Autodesk Inventor part; units mm, degrees
ref_plane "YZ Plane" through (0, 0, 0) normal (1, 0, 0) x (0, 1, 0)
ref_plane "XZ Plane" through (0, 0, 0) normal (0, 1, 0) x (-1, 0, 0)
ref_plane "XY Plane" through (0, 0, 0) normal (0, 0, 1) x (1, 0, 0)
sketch "Sketch1" plane through (0, 0, 0) normal (0, 1, 0) x (-1, 0, 0)
  line L0 (0, 0) -> (-25, 0)
  line L1 (-25, 0) -> (-25, -46.5)
  line L2 (-25, -46.5) -> (0, -46.5)
  line L3 (0, -46.5) -> (0, 0)
  dimension "d0" = 25
  dimension "d1" = 46.5
extrude "Extrusion1" add sketch "Sketch1" along normal blind 2
sketch "Sketch2" plane through (0, 2, 0) normal (0, 1, 0) x (1, 0, 0)
  line L0 (25, 46.5) -> (0, 46.5)
  line L1 (0, 46.5) -> (6, 46.5)
  line L2 (6, 46.5) -> (6, 36.5)
  line L3 (6, 36.5) -> (0, 36.5)
  line L4 (0, 36.5) -> (0, 46.5)
  line L5 (25, 46.5) -> (19, 46.5)
  line L6 (19, 46.5) -> (19, 36.5)
  line L7 (19, 36.5) -> (25, 36.5)
  line L8 (25, 36.5) -> (25, 46.5)
  point P0 (0, 0)
  dimension "d4" = 6
  dimension "d5" = 10
  dimension "d6" = 6
extrude "Extrusion2" add sketch "Sketch2" along normal blind 3
sketch "Sketch4" plane through (0, 2, 0) normal (0, 1, 0) x (1, 0, 0)
  line L0 (0, 0) -> (25, 0)
  line L1 (25, 0) -> (25, 36.5)
  point P0 (12.5, 4)
  dimension "d18" = 4
  dimension "d19" = 12.5
hole "Hole2" at (12.5, 2, -4) direction (0, -1, 0) diameter 3.2 end through all
properties part number "mlx_mount_3mm"
For this review, take the finished solid that the model builds, in its own axes (mm). A direction names the side the tool comes from. Round coordinates to 2 decimals unless told otherwise and drop trailing zeros. Write each loop counter-clockwise with the first axis right and the second up, starting at its lowest first coordinate (ties: lowest second). Pieces come first, ordered by that corner, then holes. Notation, with made-up numbers: (22.25, 24.5) -> (43.25, 24.5) arc R26 ccw to (43.25, 63.5) -> close; hole circle Ø8 at (76.25, 88.5). An arc over 180 degrees is marked (long way). One line per question, with ' | ' between items. Start each with the question number.
1) Machinability: for faces 1 (the flat face through (22, 3, -36.5)), 2 (the flat face through (12, 1, 0)), 3 (the flat face through (19, 3, -42)), which of the approach directions +Z, -Z, +X, -X, +Y, -Y give a long, thin tool a straight path to every point of the face, cutting with its end or side? Answer none if there is none.
2) Add section A-A (x = 12.5). Write out the cut boundary in (y, z).
3) Wall thickness on line 1 along X through (y, z) = (2.8, -42); line 2 along Z through (x, y) = (12.5, 1); line 3 along X through (y, z) = (0.7, -4): over which ranges is each line inside the solid? List them lowest first.
4) Add section C-C (z = -42.5). Write out the cut boundary in (x, y).
5) Add section D-D (x = 20). Write out the cut boundary in (y, z).
6) For pin 1 Ø3 at (y, z) = (3, -12) entering from -X; pin 2 Ø1.9 at (x, z) = (12.5, -4) entering from -Y; pin 3 Ø1.5 at (x, y) = (23, 4) entering from +Z, all flat-tipped, find the tip position at first contact; note any pin that passes through.
7) Mouldability with a two-part tool opening along X and no side actions: class faces 4 (the flat face through (13, 1, -46.5)), 5 (the flat face through (0, 1, -29)), 6 (the flat face through (6, 3, -42)) as +X half, -X half, draft (parallel to the pull), parting line (faces both ways), or undercut.
8) Add section B-B (z = -4). Write out the cut boundary in (x, y).
Reported:
1) face 1: +Z, +X, -X, +Y | face 2: +Z, +X, -X, +Y, -Y | face 3: +Z, -Z, +Y
2) outline: (0, -46.5) -> (2, -46.5) -> (2, -5.6) -> (0, -5.6) -> close; (0, -2.4) -> (2, -2.4) -> (2, 0) -> (0, 0) -> close
3) line 1: x = 0 to 6, 19 to 25 | line 2: z = -46.5 to -5.6, -2.4 to 0 | line 3: x = 0 to 10.9, 14.1 to 25
4) outline: (0, 0) -> (25, 0) -> (25, 5) -> (19, 5) -> (19, 2) -> (6, 2) -> (6, 5) -> (0, 5) -> close
5) outline: (0, -46.5) -> (5, -46.5) -> (5, -36.5) -> (2, -36.5) -> (2, 0) -> (0, 0) -> close
6) pin 1: stops at x = 0 | pin 2: passes through | pin 3: stops at z = -36.5
7) face 4: draft | face 5: -X half | face 6: undercut
8) outline: (0, 0) -> (10.9, 0) -> (10.9, 2) -> (0, 2) -> close; (14.1, 0) -> (25, 0) -> (25, 2) -> (14.1, 2) -> close
